Check sheet for the modelled part. Datum: model origin and axes. Units: mm. A direction names the side the tool comes from. Round coordinates to 2 decimals unless told otherwise and drop trailing zeros. Write each loop counter-clockwise with the first axis right and the second up, starting at its lowest first coordinate (ties: lowest second). Pieces come first, ordered by that corner, then holes. Notation, with made-up numbers: (30.5, 26.25) -> (86.5, 26.25) arc R29 cw to (86.5, 59.25) -> close; hole circle Ø10 at (28, 59). An arc over 180 degrees is marked (long way). Answer as a JSON object with one key per item and string values. Group by question number.
```python
from build123d import *

# Parameters (mm, degrees)
SKETCH_1_R      = 3.9
SKETCH_1_R_2    = 3.4
EXTRUDE_1_DEPTH = 100


with BuildPart() as part:
    # 草图1 → 凸台-拉伸1 (new body)
    with BuildSketch(Plane.XY):
        with BuildLine():
            Line((-24.732808051, 19.848597475), (-40.482808051, 19.848597475))
            Line((-40.482808051, 19.848597475), (-40.482808051, 4.098597475))
            Line((-40.482808051, 4.098597475), (-37.482808051, 4.098597475))
            Line((-37.482808051, 4.098597475), (-37.482808051, 7.048597475))
            Line((-37.482808051, 7.048597475), (-29.482808051, 7.048597475))
            Line((-29.482808051, 7.048597475), (-29.482808051, 5.044749898))
            ThreePointArc((-29.482808051, 5.044749898), (-26.482808051, -0.151402525), (-29.482808051, -5.347554947))
            Line((-29.482808051, -5.347554947), (-29.482808051, -7.351402525))
            Line((-29.482808051, -7.351402525), (-37.482808051, -7.351402525))
            Line((-37.482808051, -7.351402525), (-37.482808051, -4.401402525))
            Line((-37.482808051, -4.401402525), (-40.482808051, -4.401402525))
            Line((-40.482808051, -4.401402525), (-40.482808051, -20.151402525))
            Line((-40.482808051, -20.151402525), (-24.732808051, -20.151402525))
            Line((-24.732808051, -20.151402525), (-24.732808051, -17.151402525))
            Line((-24.732808051, -17.151402525), (-27.682808051, -17.151402525))
            Line((-27.682808051, -17.151402525), (-27.682808051, -9.151402525))
            Line((-27.682808051, -9.151402525), (-25.678960473, -9.151402525))
            ThreePointArc((-25.678960473, -9.151402525), (-20.482808051, -6.151402525), (-15.286655628, -9.151402525))
            Line((-15.286655628, -9.151402525), (-13.282808051, -9.151402525))
            Line((-13.282808051, -9.151402525), (-13.282808051, -17.151402525))
            Line((-13.282808051, -17.151402525), (-16.232808051, -17.151402525))
            Line((-16.232808051, -17.151402525), (-16.232808051, -20.151402525))
            Line((-16.232808051, -20.151402525), (-0.482808051, -20.151402525))
            Line((-0.482808051, -20.151402525), (15.267191949, -20.151402525))
            Line((15.267191949, -20.151402525), (15.267191949, -17.151402525))
            Line((15.267191949, -17.151402525), (12.317191949, -17.151402525))
            Line((12.317191949, -17.151402525), (12.317191949, -9.151402525))
            Line((12.317191949, -9.151402525), (14.321039527, -9.151402525))
            ThreePointArc((14.321039527, -9.151402525), (19.517191949, -6.151402525), (24.713344372, -9.151402525))
            Line((24.713344372, -9.151402525), (26.717191949, -9.151402525))
            Line((26.717191949, -9.151402525), (26.717191949, -17.151402525))
            Line((26.717191949, -17.151402525), (23.767191949, -17.151402525))
            Line((23.767191949, -17.151402525), (23.767191949, -20.151402525))
            Line((23.767191949, -20.151402525), (39.517191949, -20.151402525))
            Line((39.517191949, -20.151402525), (39.517191949, -4.401402525))
            Line((39.517191949, -4.401402525), (36.517191949, -4.401402525))
            Line((36.517191949, -4.401402525), (36.517191949, -7.351402525))
            Line((36.517191949, -7.351402525), (28.517191949, -7.351402525))
            Line((28.517191949, -7.351402525), (28.517191949, -5.347554947))
            ThreePointArc((28.517191949, -5.347554947), (25.517191949, -0.151402525), (28.517191949, 5.044749898))
            Line((28.517191949, 5.044749898), (28.517191949, 7.048597475))
            Line((28.517191949, 7.048597475), (36.517191949, 7.048597475))
            Line((36.517191949, 7.048597475), (36.517191949, 4.098597475))
            Line((36.517191949, 4.098597475), (39.517191949, 4.098597475))
            Line((39.517191949, 4.098597475), (39.517191949, 19.848597475))
            Line((39.517191949, 19.848597475), (23.767191949, 19.848597475))
            Line((23.767191949, 19.848597475), (23.767191949, 16.848597475))
            Line((23.767191949, 16.848597475), (26.717191949, 16.848597475))
            Line((26.717191949, 16.848597475), (26.717191949, 8.848597475))
            Line((26.717191949, 8.848597475), (24.713344372, 8.848597475))
            ThreePointArc((24.713344372, 8.848597475), (19.517191949, 5.848597475), (14.321039527, 8.848597475))
            Line((14.321039527, 8.848597475), (12.317191949, 8.848597475))
            Line((12.317191949, 8.848597475), (12.317191949, 16.848597475))
            Line((12.317191949, 16.848597475), (15.267191949, 16.848597475))
            Line((15.267191949, 16.848597475), (15.267191949, 19.848597475))
            Line((15.267191949, 19.848597475), (-0.482808051, 19.848597475))
            Line((-0.482808051, 19.848597475), (-16.232808051, 19.848597475))
            Line((-16.232808051, 19.848597475), (-16.232808051, 16.848597475))
            Line((-16.232808051, 16.848597475), (-13.282808051, 16.848597475))
            Line((-13.282808051, 16.848597475), (-13.282808051, 8.848597475))
            Line((-13.282808051, 8.848597475), (-15.286655628, 8.848597475))
            ThreePointArc((-15.286655628, 8.848597475), (-20.482808051, 5.848597475), (-25.678960473, 8.848597475))
            Line((-25.678960473, 8.848597475), (-27.682808051, 8.848597475))
            Line((-27.682808051, 8.848597475), (-27.682808051, 16.848597475))
            Line((-27.682808051, 16.848597475), (-24.732808051, 16.848597475))
            Line((-24.732808051, 16.848597475), (-24.732808051, 19.848597475))
        make_face()
        with Locations((-34.082808051, 13.448597475)):
            Circle(SKETCH_1_R, mode=Mode.SUBTRACT)
        with Locations((-34.082808051, -13.751402525)):
            Circle(SKETCH_1_R, mode=Mode.SUBTRACT)
        with Locations((-20.482808051, -0.151402525)):
            Circle(SKETCH_1_R_2, mode=Mode.SUBTRACT)
        with Locations((33.117191949, 13.448597475)):
            Circle(SKETCH_1_R, mode=Mode.SUBTRACT)
        with Locations((33.117191949, -13.751402525)):
            Circle(SKETCH_1_R, mode=Mode.SUBTRACT)
        with Locations((19.517191949, -0.151402525)):
            Circle(SKETCH_1_R_2, mode=Mode.SUBTRACT)
        with BuildLine():
            Line((-10.082808051, 15.048597475), (-10.082808051, 5.631330393))
            ThreePointArc((-10.082808051, 5.631330393), (-14.482808051, -0.151402525), (-10.082808051, -5.934135442))
            Line((-10.082808051, -5.934135442), (-10.082808051, -15.351402525))
            ThreePointArc((-10.082808051, -15.351402525), (-9.789914832, -16.058509306), (-9.082808051, -16.351402525))
            Line((-9.082808051, -16.351402525), (8.117191949, -16.351402525))
            ThreePointArc((8.117191949, -16.351402525), (8.824298731, -16.058509306), (9.117191949, -15.351402525))
            Line((9.117191949, -15.351402525), (9.117191949, -5.934135442))
            ThreePointArc((9.117191949, -5.934135442), (13.517191949, -0.151402525), (9.117191949, 5.631330393))
            Line((9.117191949, 5.631330393), (9.117191949, 15.048597475))
            ThreePointArc((9.117191949, 15.048597475), (8.824298731, 15.755704257), (8.117191949, 16.048597475))
            Line((8.117191949, 16.048597475), (-9.082808051, 16.048597475))
            ThreePointArc((-9.082808051, 16.048597475), (-9.789914832, 15.755704257), (-10.082808051, 15.048597475))
        make_face(mode=Mode.SUBTRACT)
    extrude(amount=EXTRUDE_1_DEPTH)


solid = part.part
```
(1) Section check C-C on x = -33.5. Record the cut outline in (y, z), then the cut area to 3 significant figures.
(2) Section check D-D on y = 1. Record the cut outline in (x, z), then the cut area to 3 significant figures.
(3) Section check A-A on x = -3.5. Record the cut outline in (y, z).
(4) Section check B-B on y = -11.5. Record the cut outline in (x, z).
(5) Access from +Z, -Z, +X, -X, +Y, -Y to the whole of each face (thin tool, end or side, straight path). Record for faces 5 (the flat face through (38, -4.401, 49)), 6 (the flat face through (14, -17.151, 49)), 7 (the flat face through (-16.233, -19, 49)), 8 (the flat face through (-33, -20.151, 49)), 9 (the flat face through (23.767, 18, 49)).
(6) Release check for a two-part mould opening along Y. For faces 1 (the flat face through (-1, -20.151, 49)), 2 (the flat face through (36.517, 6, 49)), 3 (the flat face through (-24.733, -19, 49)), 4 (the flat face through (-37.483, -6, 49)) record: pulls with the +Y half, pulls with the -Y half, needs draft (parallel to the pull), parting line crosses it, or undercut.
(7) Scan lines: line 1 along X through (y, z) = (9, 9.5); line 2 along Y through (x, z) = (25, 95); line 3 along Y through (x, z) = (5.5, 49.5). Record each from-to range of solid material in increasing order.
(8) Go/stop test with flat-tipped pins: pin 1 Ø3 at (x, z) = (-20.5, 67.5) entering from -Y; pin 2 Ø1 at (y, z) = (0.5, 56.5) entering from -X. Record where each tip stops, or that it passes through.
Data:
{
 "1": {"outline": "(-20.15, 0) -> (-17.61, 0) -> (-17.61, 100) -> (-20.15, 100) -> close; (-9.9, 0) -> (-7.35, 0) -> (-7.35, 100) -> (-9.9, 100) -> close; (7.05, 0) -> (9.59, 0) -> (9.59, 100) -> (7.05, 100) -> close; (17.3, 0) -> (19.85, 0) -> (19.85, 100) -> (17.3, 100) -> close", "area": "1,020 mm²"},
 "2": {"outline": "(-26.59, 0) -> (-23.68, 0) -> (-23.68, 100) -> (-26.59, 100) -> close; (-17.28, 0) -> (-14.37, 0) -> (-14.37, 100) -> (-17.28, 100) -> close; (13.41, 0) -> (16.32, 0) -> (16.32, 100) -> (13.41, 100) -> close; (22.72, 0) -> (25.63, 0) -> (25.63, 100) -> (22.72, 100) -> close", "area": "1,160 mm²"},
 "3": {"outline": "(-20.15, 0) -> (-16.35, 0) -> (-16.35, 100) -> (-20.15, 100) -> close; (16.05, 0) -> (19.85, 0) -> (19.85, 100) -> (16.05, 100) -> close"},
 "4": {"outline": "(-40.48, 0) -> (-37.27, 0) -> (-37.27, 100) -> (-40.48, 100) -> close; (-30.9, 0) -> (-27.68, 0) -> (-27.68, 100) -> (-30.9, 100) -> close; (-13.28, 0) -> (-10.08, 0) -> (-10.08, 100) -> (-13.28, 100) -> close; (9.12, 0) -> (12.32, 0) -> (12.32, 100) -> (9.12, 100) -> close; (26.72, 0) -> (29.93, 0) -> (29.93, 100) -> (26.72, 100) -> close; (36.3, 0) -> (39.52, 0) -> (39.52, 100) -> (36.3, 100) -> close"},
 "5": {"face 5": "+Z, -Z, +X", "face 6": "+Z, -Z", "face 7": "+Z, -Z, -Y", "face 8": "+Z, -Z, +X, -X, -Y", "face 9": "+Z, -Z, +Y"},
 "6": {"face 1": "pulls with the -Y half", "face 2": "undercut", "face 3": "needs draft", "face 4": "undercut"},
 "7": {"line 1": "x = -40.48 to -27.68, -13.28 to -10.08, 9.12 to 12.32, 26.72 to 39.52", "line 2": "y = -20.15 to -17.15, -9.15 to 8.85, 16.85 to 19.85", "line 3": "y = -20.15 to -16.35, 16.05 to 19.85"},
 "8": {"pin 1": "stops at y = -6.35", "pin 2": "stops at x = -26.59"}
}
